from build123d import *

# Parameters (mm, degrees)
F0_W     = 25.4
F0_H     = 25.4
F0_R     = 4.7625
F0_W_2   = 3.175
F0_W_3   = 6.35
F0_R_2   = 2.54
F1_DEPTH = 14.2875
F2_DEPTH = 19.05
F3_DEPTH = 5.08
F4_DEPTH = 14.2875
F5_SIZE  = 0.63499
F6_R     = 0.635


# Not quite as in the source:
# - a fillet or chamfer is up to 0.001 mm smaller than in the source, because OpenCascade refuses the exact size
# - a feature names something its author has since deleted; it is built from what else it names


with BuildPart() as f1:
    # F0 (on Top) → F1 (new body)
    with BuildSketch(Plane.XY):
        Polygon((-6.35, 12.7), (-3.175, 12.7), (-3.175, 22.225), (-41.275, 22.225), (-41.275, -22.225), (-3.175, -22.225), (-3.175, -12.7), (-6.35, -12.7), (-31.75, -12.7), (-31.75, 12.7), align=None)
        with Locations((-19.05, 0)):
            Rectangle(F0_W, F0_H)
        with Locations((-19.05, 0)):
            Circle(F0_R, mode=Mode.SUBTRACT)
        with Locations((-4.7625, 0)):
            Rectangle(F0_W_2, F0_H)
        Rectangle(F0_W_3, F0_H)
        Polygon((3.175, 12.7), (3.175, 22.225), (2.54, 22.225), (-2.54, 22.225), (-3.175, 22.225), (-3.175, 12.7), align=None)
        with Locations((0, 15.875)):
            Circle(F0_R_2, mode=Mode.SUBTRACT)
        Polygon((2.54, -22.225), (3.175, -22.225), (3.175, -12.7), (-3.175, -12.7), (-3.175, -22.225), (-2.54, -22.225), align=None)
        with Locations((0, -15.875)):
            Circle(F0_R_2, mode=Mode.SUBTRACT)
        Polygon((41.275, -22.225), (41.275, 22.225), (3.175, 22.225), (3.175, 12.7), (6.35, 12.7), (31.75, 12.7), (31.75, -12.7), (6.35, -12.7), (3.175, -12.7), (3.175, -22.225), align=None)
        with Locations((4.7625, 0)):
            Rectangle(F0_W_2, F0_H)
        with Locations((19.05, 0)):
            Rectangle(F0_W, F0_H)
        with Locations((19.05, 0)):
            Circle(F0_R, mode=Mode.SUBTRACT)
        with Locations((19.05, 0)):
            Circle(F0_R)
        with Locations((-19.05, 0)):
            Circle(F0_R)
    extrude(amount=-F1_DEPTH)

    # F0 (on Top) → F2 (join)
    with BuildSketch(Plane.XY):
        with Locations((-19.05, 0)):
            Rectangle(F0_W, F0_H)
        with Locations((-19.05, 0)):
            Circle(F0_R, mode=Mode.SUBTRACT)
        with Locations((19.05, 0)):
            Rectangle(F0_W, F0_H)
        with Locations((19.05, 0)):
            Circle(F0_R, mode=Mode.SUBTRACT)
    extrude(amount=F2_DEPTH)

    # F0 (on Top) → F3 (cut)
    with BuildSketch(Plane.XY):
        Rectangle(F0_W_3, F0_H)
        Polygon((2.54, -22.225), (3.175, -22.225), (3.175, -12.7), (-3.175, -12.7), (-3.175, -22.225), (-2.54, -22.225), align=None)
        with Locations((0, -15.875)):
            Circle(F0_R_2, mode=Mode.SUBTRACT)
        Polygon((3.175, 12.7), (3.175, 22.225), (2.54, 22.225), (-2.54, 22.225), (-3.175, 22.225), (-3.175, 12.7), align=None)
        with Locations((0, 15.875)):
            Circle(F0_R_2, mode=Mode.SUBTRACT)
    extrude(amount=-F3_DEPTH, mode=Mode.SUBTRACT)

    # F0 (on Top) → F4 (cut)
    with BuildSketch(Plane.XY):
        with Locations((0, -15.875)):
            Circle(F0_R_2)
        with Locations((0, 15.875)):
            Circle(F0_R_2)
    extrude(amount=-F4_DEPTH, mode=Mode.SUBTRACT)

    # F5 (size 0.635 in the source; OpenCascade refuses exactly that, so slightly less here)
    f5_edges = [f1.edges().sort_by_distance(p)[0] for p in [
        (3.175, 0, -5.08),
        (-3.175, 0, -5.08),
        (3.175, 0, 0),
        (-3.175, 0, 0),
    ]]
    chamfer(f5_edges, length=F5_SIZE)

    # F6
    f6_edges = [f1.edges().sort_by_distance(p)[0] for p in [
        (-22.542495, -22.225, 0),
        (-3.492495, -22.225, -0.317495),
        (-2.857505, -22.225, -4.762505),
        (0, -22.225, -5.08),
        (2.857505, -22.225, -4.762505),
        (3.175, -22.225, -2.54),
        (3.492495, -22.225, -0.317495),
        (22.542495, -22.225, 0),
        (-41.275, -22.225, -7.14375),
        (-41.275, 0, 0),
        (-41.275, 22.225, -7.14375),
        (-22.542495, 22.225, 0),
        (-3.175, 22.225, -2.54),
        (-3.492495, 22.225, -0.317495),
        (0, 22.225, -5.08),
        (-2.857505, 22.225, -4.762505),
        (22.542495, 22.225, 0),
        (3.175, 22.225, -2.54),
        (3.492495, 22.225, -0.317495),
        (41.275, 22.225, -7.14375),
        (41.275, 0, 0),
        (41.275, -22.225, -7.14375),
        (2.857505, 22.225, -4.762505),
        (-3.175, -22.225, -2.54),
    ]]
    fillet(f6_edges, radius=F6_R)


solid = f1.part
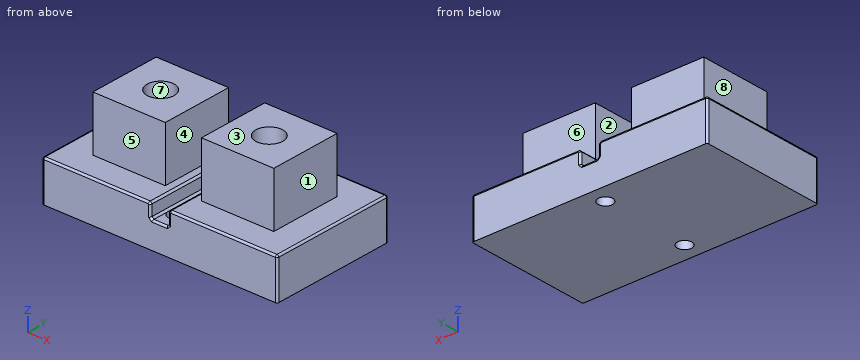
Read the model definition and answer for the solid it produces. Units are mm, in the model's axes. Face numbers are marked on the shaded views. A direction names the side the tool comes from. Round coordinates to 2 decimals unless told otherwise and drop trailing zeros. Loops run counter-clockwise (first coordinate to the right, second up) from the corner with the lowest first, then second, coordinate; pieces in that order, holes last.
Q1. Section A-A on x = 0 is taken. Write down the section's boundary in (y, z) (1 decimal).
Q2. Determine the mould class of the marked faces 1, 2 and 3 for opening direction X: released by +X, released by -X, zero draft, split by the parting line, or undercut.
Q3. Consider probe 1 along Y at (x, z) = (0, -11) (3 decimals); probe 2 along X at (y, z) = (9, 7); probe 3 along X at (y, z) = (-5, -3.5) (3 decimals). Determine where each line is inside the solid, lowest interval first.
Q4. Which of the six approach directions +Z, -Z, +X, -X, +Y, -Y give full straight-line access (tool end or side, diameter ignored) to the marked faces 4, 5, 6, 7 and 8?
Q5. Section B-B on z = 17 is taken. Give the number of separate pieces and of enclosed holes in the cut face, and give its area (3 significant figures).
Q6. Each of these flat-tipped pins is pushed along its axis until it touches: pin 1 (15 mm diameter, centred on y = -2.5, z = 10, fed in from +X); pin 2 (3 mm diameter, centred on x = -20, y = 1.5, fed in from +Z); pin 3 (2 mm diameter, centred on x = -15, z = 12, fed in from -Y); pin 4 (10 mm diameter, centred on x = 0, z = 10, fed in from +Y). Where does it stop, or does it pass through?
Output:
1. outline: (-22.2, -14.3) - (-18.4, -14.3) - (-18.4, -5.1) - (-21.6, -5.1) arc R0.6 ccw to (-22.2, -5.7) - close; (-13.3, -14.3) - (13.3, -14.3) - (13.3, -5.1) - (-13.3, -5.1) - close; (18.4, -14.3) - (22.2, -14.3) - (22.2, -5.7) arc R0.6 ccw to (21.6, -5.1) - (18.4, -5.1) - close
2. face 1: released by +X
2. face 2: undercut
2. face 3: zero draft
3. probe 1: y = -22.225 to -18.415, -13.335 to 13.335, 18.415 to 22.225
3. probe 2: x = -31.75 to -6.35, 6.35 to 31.75
3. probe 3: x = -41.275 to -3.175, 3.175 to 41.275
4. face 4: +Z, +Y, -Y
4. face 5: +Z, +X, -X, -Y
4. face 6: +Z, +X, -X, +Y
4. face 7: +Z
4. face 8: +Z, -X, +Y, -Y
5. separate pieces: 2
5. enclosed holes: 2
5. area: 1,150 mm2
6. pin 1: stops at x = 31.75
6. pin 2: stops at z = 0
6. pin 3: stops at y = -12.7
6. pin 4: passes through
